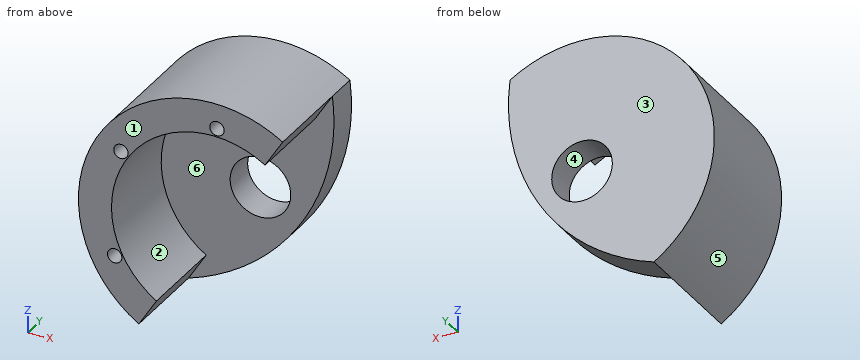
```python
from build123d import *

# Parameters (mm, degrees)
EXTRUDE_2_DEPTH     = 17
EXTRUDE_3_DEPTH     = 6
SKETCH_5_R          = 4.5
CUT_EXTRUDE_1_DEPTH = 6
SKETCH_7_R          = 1.3
CUT_EXTRUDE_2_DEPTH = 10
SKETCH1_R           = 5.5
CUT_EXTRUDE1_DEPTH  = 38.960505792
CUT_EXTRUDE_3_REACH = 39.961
SKETCH_10_R         = 18


with BuildPart() as part:
    # 草图2 → 凸台-拉伸2 (new body)
    with BuildSketch(Plane(origin=(0, 0, 0), x_dir=(1, 0, 0), z_dir=(0, 1, 0))):
        with BuildLine():
            Line((-13.050585614, 20.141554437), (-8.239089232, 12.534648325))
            ThreePointArc((-8.239089232, 12.534648325), (-12.534648325, -8.239089232), (8.239089232, -12.534648325))
            Line((8.239089232, -12.534648325), (13.050585614, -20.141554437))
            ThreePointArc((13.050585614, -20.141554437), (-20.141554437, -13.050585614), (-13.050585614, 20.141554437))
        make_face()
    extrude(amount=EXTRUDE_2_DEPTH)

    # 草图4 → 凸台-拉伸3 (add)
    with BuildSketch(Plane(origin=(0, 17, 0), x_dir=(1, 0, 0), z_dir=(0, 1, 0))):
        with BuildLine():
            ThreePointArc((13.050585614, -20.141554437), (-20.141554437, -13.050585614), (-13.050585614, 20.141554437))
            ThreePointArc((-13.050585614, 20.141554437), (7.331987605, 4.750712377), (13.050585614, -20.141554437))
        make_face()
    extrude(amount=EXTRUDE_3_DEPTH)

    # 草图5 → 切除-拉伸1 (cut)
    with BuildSketch(Plane(origin=(0, 23, 0), x_dir=(1, 0, 0), z_dir=(0, 1, 0))):
        with Locations(Location((0, 0, 0), (0, 0, 270))):
            Circle(SKETCH_5_R)
    extrude(amount=-CUT_EXTRUDE_1_DEPTH, mode=Mode.SUBTRACT)

    # 草图7 → 切除-拉伸2 (cut)
    with BuildSketch(Plane.XZ):
        with Locations(Location((-17.423360164, -8.756513039, 0), (0, 0, 270))):
            Circle(SKETCH_7_R)
        with Locations(Location((-16.295042822, 10.710816001, 0), (0, 0, 270))):
            Circle(SKETCH_7_R)
        with Locations(Location((1.128317341, 19.467329041, 0), (0, 0, 270))):
            Circle(SKETCH_7_R)
    extrude(amount=-CUT_EXTRUDE_2_DEPTH, mode=Mode.SUBTRACT)

    # Sketch1 → Cut-Extrude1 (cut, through all)
    with BuildSketch(Plane.XZ.offset(-17)):
        with Locations(Location((0, 0, 0), (0, 0, 270))):
            Circle(SKETCH1_R)
    extrude(amount=-CUT_EXTRUDE1_DEPTH, mode=Mode.SUBTRACT)

    # 草图10 → 切除-拉伸3 (cut, up to next)
    with BuildSketch(Plane.XZ.offset(-17), mode=Mode.PRIVATE) as cut_extrude_3_sk1:
        Circle(SKETCH_10_R)
    cut_extrude_3_tool1 = extrude(cut_extrude_3_sk1.sketch, amount=CUT_EXTRUDE_3_REACH, mode=Mode.PRIVATE) & part.part
    add(cut_extrude_3_tool1.solids().sort_by_distance((0, 17, 0))[0], mode=Mode.SUBTRACT)


solid = part.part
```
The model under review builds one solid part; all positions refer to its coordinate system, in mm. Face numbers are marked on the shaded views. A direction names the side the tool comes from. Round coordinates to 2 decimals unless told otherwise and drop trailing zeros. Order: outer loops, then holes, each group sorted by start corner. A loop starts at its lowest first (then second) coordinate and runs counter-clockwise, first axis right, second up. Notation, with made-up numbers: M -32.5,12.5 L 21.5,12.5 A8 ccw 21.5,16.5 Z; hole C 53.5,49.25 d11. An arc over 180 degrees is marked long. Use a Markdown table: item, result.
1) Wall thickness on line 1 along Y through (x, z) = (-15.5, -3.5); line 2 along Z through (x, y) = (-13.5, 6); line 3 along X through (y, z) = (3, 19): over which ranges is each line inside the solid? List them lowest first. Write a range as [from, to].
Report:
| item | result |
|---|---|
| line 1 | [17, 23] |
| line 2 | [-19.84, -11.91], [11.91, 19.84] |
| line 3 | [-14.66, -0.08], [2.34, 12.33] |
2) Draft analysis for pull direction Z (two halves, no side actions). For the marked faces 3, 4, 5 and 6, state which applies: released by +Z, released by -Z, zero draft, split by the parting line, or undercut.
Report:
| item | result |
|---|---|
| face 3 | zero draft |
| face 4 | undercut |
| face 5 | split by the parting line |
| face 6 | undercut |
3) Insertion check: pin 1 (1 mm diameter, centred on x = 7.5, y = 8.5, fed in from +Z); pin 2 (1.3 mm diameter, centred on x = -16.5, z = 10.5, fed in from -Y); pin 3 (4 mm diameter, centred on y = 11, z = -1, fed in from +X). Each pin has a flat end and moves straight along its axis. Give the tip position at first contact, or say it passes through.
Report:
| item | result |
|---|---|
| pin 1 | z = 22.96 |
| pin 2 | y = 10 |
| pin 3 | x = -17.75 |
4) Tool access review of the marked faces 1 and 2: name each direction out of +Z, -Z, +X, -X, +Y, -Y from which nothing blocks a thin tool from reaching the whole face with its end or side.
Report:
| item | result |
|---|---|
| face 1 | +Z, -Z, +X, -X, -Y |
| face 2 | -Y |
5) Consider section C-C (z = 11.5). Write out the cut boundary in (x, y).
Report:
| item | result |
|---|---|
| outline | M -21.07,0 L -17.33,0 L -17.33,10 L -15.26,10 L -15.26,0 L -13.85,0 L -13.85,17 L 13.11,17 L 13.11,23 L -21.07,23 Z |
6) Consider section A-A (z = 0). Write out the cut boundary in (x, y), then the cut area to 3 significant figures.
Report:
| item | result |
|---|---|
| outline | M -24,0 L -18,0 L -18,17 L -5.5,17 L -5.5,23 L -24,23 Z; M 5.5,17 L 9.94,17 L 9.94,23 L 5.5,23 Z |
| area | 240 mm^2 |
